```python
from build123d import *

# Parameters (mm, degrees)
F0_W     = 35
F0_H     = 28
F1_DEPTH = 14
F3_D     = 12.7
F4_DEPTH = 6.5
F5_D     = 3
F6_DEPTH = 1.5
F7_R     = 5


with BuildPart() as f1:
    # F0 (on Top) → F1 (new body)
    with BuildSketch(Plane.XY):
        Rectangle(F0_W, F0_H)
    extrude(amount=F1_DEPTH)

    # F3 (through all)
    with Locations(Plane(origin=(-17.5, 0, 0), x_dir=(0, -1, 0), z_dir=(-1, 0, 0))):
        with Locations((0, 7)):
            Hole(F3_D / 2)

    # F4 (cut): a face of the model
    f4_faces = [f1.faces().sort_by_distance(p)[0] for p in [
        (0, 0, 14),
    ]]
    extrude(f4_faces, amount=-F4_DEPTH, mode=Mode.SUBTRACT)

    # F5 (through all)
    with Locations(Plane(origin=(0, 0, 0), x_dir=(1, 0, 0), z_dir=(0, 0, -1))):
        with Locations((10.9, -10.2), (-10.9, -10.2), (-10.9, 10.2), (10.9, 10.2)):
            Hole(F5_D / 2)

    # F6 (add): a face of the model
    f6_faces = [f1.faces().sort_by_distance(p)[0] for p in [
        (0, 0, 0),
    ]]
    extrude(f6_faces, amount=F6_DEPTH)

    # F7
    f7_edges = [f1.edges().sort_by_distance(p)[0] for p in [
        (-17.5, -14, 3),
        (-17.5, 14, 3),
        (17.5, 14, 3),
        (17.5, -14, 3),
    ]]
    fillet(f7_edges, radius=F7_R)


solid = f1.part
```
The model under review builds one solid part; all positions refer to its coordinate system, in mm. Round coordinates to 2 decimals unless told otherwise and drop trailing zeros. Loops run counter-clockwise (first coordinate to the right, second up) from the corner with the lowest first, then second, coordinate; pieces in that order, holes last. Notation, with made-up numbers: (-17.5, 52.25) -> (15.5, 52.25) arc R19 ccw to (15.5, 79.25) -> close; hole circle Ø1 at (18, -25.5). An arc over 180 degrees is marked (long way). Answer as a JSON object with one key per item and string values. Group by question number.
1) For line 1 (Y direction, x = 10.9, z = 0.5); line 2 (Y direction, x = -10.9, z = 3); line 3 (Y direction, x = 10.9, z = 3.75), list the stretches that pass through material, from the lowest coordinate up. Write a range as [from, to].
2) For pin 1 Ø10 at (x, y) = (2, 5) entering from +Z; pin 2 Ø2.5 at (x, y) = (10.9, 10.2) entering from -Z; pin 3 Ø5 at (x, y) = (0, -1.5) entering from +Z, all flat-tipped, find the tip position at first contact; note any pin that passes through.
3) We need section C-C on z = 0.25. Write out the cut boundary in (x, y).
4) We need section B-B on x = 10.9. Write out the cut boundary in (y, z), then the cut area to 3 significant figures.
5) We need section D-D on y = 10.2. Write out the cut boundary in (x, z), then the cut area to 3 significant figures.
6) We need section A-A on z = 7. Write out the cut boundary in (x, y).
Result set:
{
 "1": {"line 1": "[-14, -11.7], [-8.7, 8.7], [11.7, 14]", "line 2": "[-14, -11.7], [-8.7, -4.93], [4.93, 8.7], [11.7, 14]", "line 3": "[-14, -11.7], [-8.7, -5.46], [5.46, 8.7], [11.7, 14]"},
 "2": {"pin 1": "z = 7.5", "pin 2": "through", "pin 3": "z = 2.07"},
 "3": {"outline": "(-17.5, -9) arc R5 ccw to (-12.5, -14) -> (12.5, -14) arc R5 ccw to (17.5, -9) -> (17.5, 9) arc R5 ccw to (12.5, 14) -> (-12.5, 14) arc R5 ccw to (-17.5, 9) -> close; hole circle Ø3 at (-10.9, -10.2); hole circle Ø3 at (-10.9, 10.2); hole circle Ø3 at (10.9, -10.2); hole circle Ø3 at (10.9, 10.2)"},
 "4": {"outline": "(-14, -1.5) -> (-11.7, -1.5) -> (-11.7, 7.5) -> (-14, 7.5) -> close; (-8.7, -1.5) -> (8.7, -1.5) -> (8.7, 7.5) -> (6.33, 7.5) arc R6.35 cw (long way) to (-6.33, 7.5) -> (-8.7, 7.5) -> close; (11.7, -1.5) -> (14, -1.5) -> (14, 7.5) -> (11.7, 7.5) -> close", "area": "128 mm²"},
 "5": {"outline": "(-17.35, -1.5) -> (-12.4, -1.5) -> (-12.4, 7.5) -> (-17.35, 7.5) -> close; (-9.4, -1.5) -> (9.4, -1.5) -> (9.4, 7.5) -> (-9.4, 7.5) -> close; (12.4, -1.5) -> (17.35, -1.5) -> (17.35, 7.5) -> (12.4, 7.5) -> close", "area": "258 mm²"},
 "6": {"outline": "(-17.5, -9) arc R5 ccw to (-12.5, -14) -> (12.5, -14) arc R5 ccw to (17.5, -9) -> (17.5, -6.35) -> (-17.5, -6.35) -> close; (-17.5, 6.35) -> (17.5, 6.35) -> (17.5, 9) arc R5 ccw to (12.5, 14) -> (-12.5, 14) arc R5 ccw to (-17.5, 9) -> close; hole circle Ø3 at (-10.9, -10.2); hole circle Ø3 at (-10.9, 10.2); hole circle Ø3 at (10.9, -10.2); hole circle Ø3 at (10.9, 10.2)"}
}
